For this review, take the finished solid that the model builds, in its own axes (mm). A direction names the side the tool comes from. Give positions to 0.01 mm unless a question says otherwise; leave off trailing zeros. Loops run counter-clockwise (first coordinate to the right, second up) from the corner with the lowest first, then second, coordinate; pieces in that order, holes last.
```python
from build123d import *

# Parameters (mm, degrees)
F1_DEPTH = 7
F3_ANGLE = 120
F4_ANGLE = 240
F6_R     = 10


with BuildPart() as f1:
    # F0 (on Top) → F1 (new body)
    with BuildSketch(Plane.XY):
        with BuildLine():
            ThreePointArc((-11, 0), (-7.7781745931, 7.7781745931), (0, 11))
            Line((0, 11), (0, 15))
            ThreePointArc((0, 15), (-11, 26), (0, 37))
            Line((0, 37), (0, 40))
            Line((0, 40), (-15, 40))
            Line((-15, 40), (-15, 0))
            Line((-15, 0), (-11, 0))
        make_face()
        with BuildLine():
            ThreePointArc((0, 11), (7.7781745931, 7.7781745931), (11, 0))
            Line((11, 0), (15, 0))
            Line((15, 0), (15, 40))
            Line((15, 40), (0, 40))
            Line((0, 40), (0, 37))
            ThreePointArc((0, 37), (7.7781745931, 33.7781745931), (11, 26))
            ThreePointArc((11, 26), (7.7781745931, 18.2218254069), (0, 15))
            Line((0, 15), (0, 11))
        make_face()
    extrude(amount=F1_DEPTH)


with BuildPart() as f3_1:
    # F3: copy of F1
    add(f1.part.rotate(Axis((0, 0, 26.0697361082), (0, 0, 1)), F3_ANGLE))


with BuildPart() as f4_1:
    # F4: copy of F1
    add(f1.part.rotate(Axis((0, 0, 26.0697361082), (0, 0, 1)), F4_ANGLE))


with BuildPart() as f1_1:
    add(f1.part)

    # F5: union F4_1, F3_1
    add(f4_1.part)
    add(f3_1.part)

    # F6
    f6_edges = [f1_1.edges().sort_by_distance(p)[0] for p in [
        (15, 40, 3.5),
        (42.141016, -7.009619, 3.5),
        (27.141016, -32.990381, 3.5),
        (-27.141016, -32.990381, 3.5),
        (-42.141016, -7.009619, 3.5),
        (-15, 40, 3.5),
        (-15, 8.660254, 3.5),
        (0, -17.320508, 3.5),
        (15, 8.660254, 3.5),
    ]]
    fillet(f6_edges, radius=F6_R)


solid = f1_1.part
```
Q1. Mouldability with a two-part tool opening along X and no side actions: class faces 3 (the flat face through (11.646, -24.044, 3.451)), 4 (the cylindrical face through (11.99, 37.15, 3.55)), 5 (the flat face through (0, 40, 3)), 6 (the flat face through (-11.83, -24.15, 3.45)) as +X half, -X half, draft (parallel to the pull), parting line (faces both ways), or undercut.
Answers:
face 3: undercut
face 4: +X half
face 5: draft
face 6: undercut
Q2. For pin 1 Ø4 at (y, z) = (-2, 5) entering from +X; pin 2 Ø3.5 at (y, z) = (19.5, 3) entering from -X; pin 3 Ø4 at (x, z) = (-11.5, 5) entering from -Y, all flat-tipped, find the tip position at first contact; note any pin that passes through.
Answers:
pin 1: stops at x = 35.93
pin 2: stops at x = -15
pin 3: stops at y = -25.11
Q3. Machinability: for faces 1 (the flat face through (15, 22, 3)), 2 (the cylindrical face through (-38.17, -8.19, 3.55)), which of the approach directions +Z, -Z, +X, -X, +Y, -Y give a long, thin tool a straight path to every point of the face, cutting with its end or side? Answer none if there is none.
Answers:
face 1: +Z, -Z, +X, +Y
face 2: +Z, -Z, -X
Q4. Consider section C-C on y = -13. Give the boundary of the cut face in (x, z).
Answers:
outline: (-38.21, 0) - (-33.52, 0) - (-33.52, 7) - (-38.21, 7) - close; (-11.52, 0) - (11.52, 0) - (11.52, 7) - (-11.52, 7) - close; (33.52, 0) - (38.21, 0) - (38.21, 7) - (33.52, 7) - close
Q5. For probe 1 along X at (y, z) = (-18, 1.25); probe 2 along Y at (x, z) = (-10, 2.25); probe 3 along X at (y, z) = (-13, 3.25), list the stretches that pass through material, from the lowest coordinate up.
Answers:
probe 1: x = -35.8 to -32.31, -12.72 to 12.72, 32.31 to 35.8
probe 2: y = -23.09 to -4.58, 4.58 to 21.42, 30.58 to 38.66
probe 3: x = -38.21 to -33.52, -11.52 to 11.52, 33.52 to 38.21
Q6. Consider section B-B on z = 2. Give the boundary of the cut face in (x, y).
Answers:
outline: (-37.14, -15.67) - (-32.14, -24.33) arc R10 ccw to (-18.48, -27.99) - (-5, -20.21) arc R10 cw to (5, -20.21) - (18.48, -27.99) arc R10 ccw to (32.14, -24.33) - (37.14, -15.67) arc R10 ccw to (33.48, -2.01) - (20, 5.77) arc R10 cw to (15, 14.43) - (15, 30) arc R10 ccw to (5, 40) - (-5, 40) arc R10 ccw to (-15, 30) - (-15, 14.43) arc R10 cw to (-20, 5.77) - (-33.48, -2.01) arc R10 ccw to start; hole circle Ø22 at (-22.52, -13); hole circle Ø22 at (0, 0); hole circle Ø22 at (0, 26); hole circle Ø22 at (22.52, -13)
Q7. Consider section A-A on y = 33.5. Give the boundary of the cut face in (x, z).
Answers:
outline: (-14.37, 0) - (-8.05, 0) - (-8.05, 7) - (-14.37, 7) - close; (8.05, 0) - (14.37, 0) - (14.37, 7) - (8.05, 7) - close
Q8. Consider section D-D on x = 8. Give the boundary of the cut face in (y, z).
Answers:
outline: (-21.94, 0) - (-7.55, 0) - (-7.55, 7) - (-21.94, 7) - close; (7.55, 0) - (18.45, 0) - (18.45, 7) - (7.55, 7) - close; (33.55, 0) - (39.54, 0) - (39.54, 7) - (33.55, 7) - close
